Check sheet for the drawn part. Datum: minimum x, y, z corner. Units: mm. Coordinates: 2 decimals unless noted, no trailing zeros. Order: outer loops, then holes, each group sorted by start corner. A loop starts at its lowest first (then second) coordinate and runs counter-clockwise, first axis right, second up. Notation, with made-up numbers: M 66.5,39 L 81.5,39 A20 cw 81.5,50 Z; hole C 52.5,-34 d1. An arc over 180 degrees is marked long. Return JSON: item names as keys, results as strings. Group by question number.
Q1. Thickness scan on probe 1 along Z at (x, y) = (5, 11.5); probe 2 along X at (y, z) = (6.5, 4.75); probe 3 along X at (y, z) = (86, 6.25) (1 decimal). Record the ranges inside material, lowest first.
Q2. Section check D-D, the plane x = 42. Enter the section's corners in (y, z) (1 decimal), then the cut area to 3 significant figures.
Q3. Section check C-C, the plane z = 13. Enter the section's corners in (x, y).
Q4. Mould release check, pull along Y, two halves, no side actions. Record for the marked faces 1 and 2: pulls with the +Y half, pulls with the -Y half, needs draft (parallel to the pull), parting line crosses it, or undercut.
Q5. Section check B-B, the plane y = 59. Enter the section's corners in (x, z), then the cut area to 3 significant figures.
Q6. Go/stop test with flat-tipped pins: pin 1 Ø2 at (x, z) = (10, 5.5) entering from +Y; pin 2 Ø1 at (x, y) = (9, 43.5) entering from +Z. Record where each tip stops, or that it passes through.
Q7. Section check A-A, the plane x = 16.5. Enter the section's corners in (y, z).
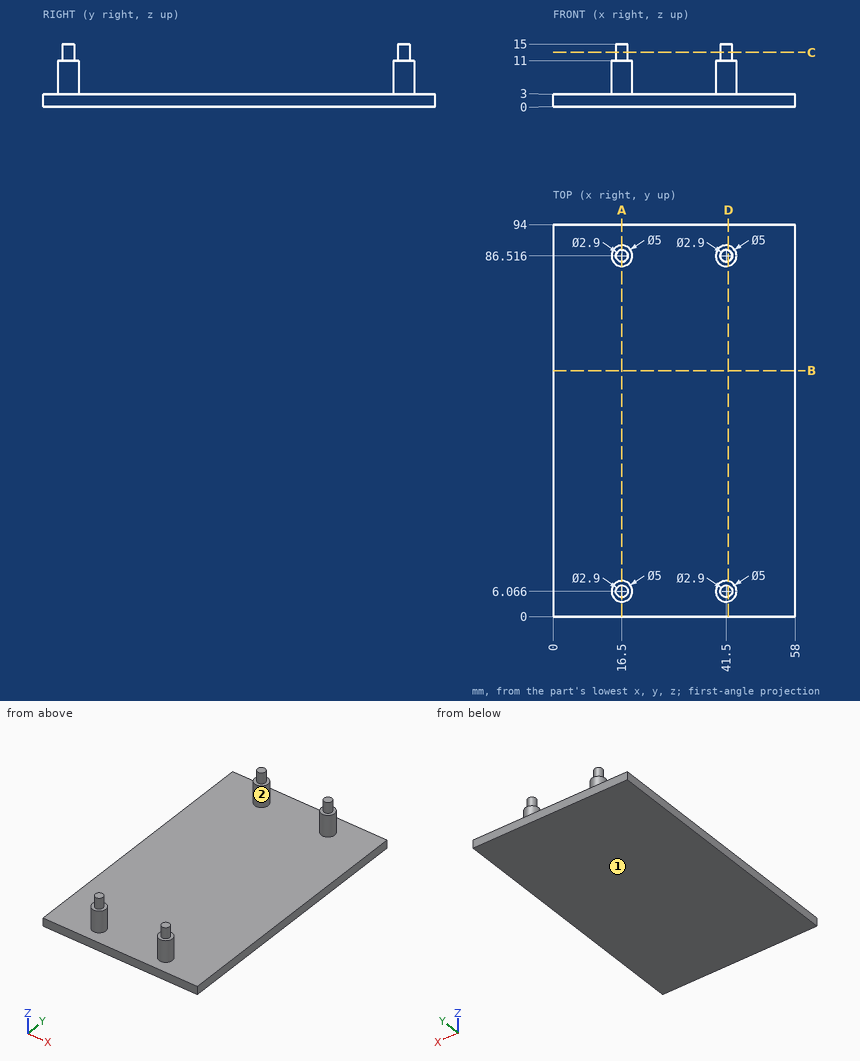
Numbers:
{
 "1": {"probe 1": "z = 0 to 3", "probe 2": "x = 14.04 to 18.96, 39.04 to 43.96", "probe 3": "x = 14.1 to 18.9, 39.1 to 43.9"},
 "2": {"outline": "M 0,0 L 94,0 L 94,3 L 89,3 L 89,11 L 87.9,11 L 87.9,15 L 85.2,15 L 85.2,11 L 84.1,11 L 84.1,3 L 8.5,3 L 8.5,11 L 7.4,11 L 7.4,15 L 4.7,15 L 4.7,11 L 3.6,11 L 3.6,3 L 0,3 Z", "area": "382 mm2"},
 "3": {"outline": "C 16.5,6.07 d2.9; C 16.5,86.52 d2.9; C 41.5,6.07 d2.9; C 41.5,86.52 d2.9"},
 "4": {"face 1": "needs draft", "face 2": "undercut"},
 "5": {"outline": "M 0,0 L 58,0 L 58,3 L 0,3 Z", "area": "174 mm2"},
 "6": {"pin 1": "passes through", "pin 2": "stops at z = 3"},
 "7": {"outline": "M 0,0 L 94,0 L 94,3 L 89.02,3 L 89.02,11 L 87.97,11 L 87.97,15 L 85.07,15 L 85.07,11 L 84.02,11 L 84.02,3 L 8.57,3 L 8.57,11 L 7.52,11 L 7.52,15 L 4.62,15 L 4.62,11 L 3.57,11 L 3.57,3 L 0,3 Z"}
}
